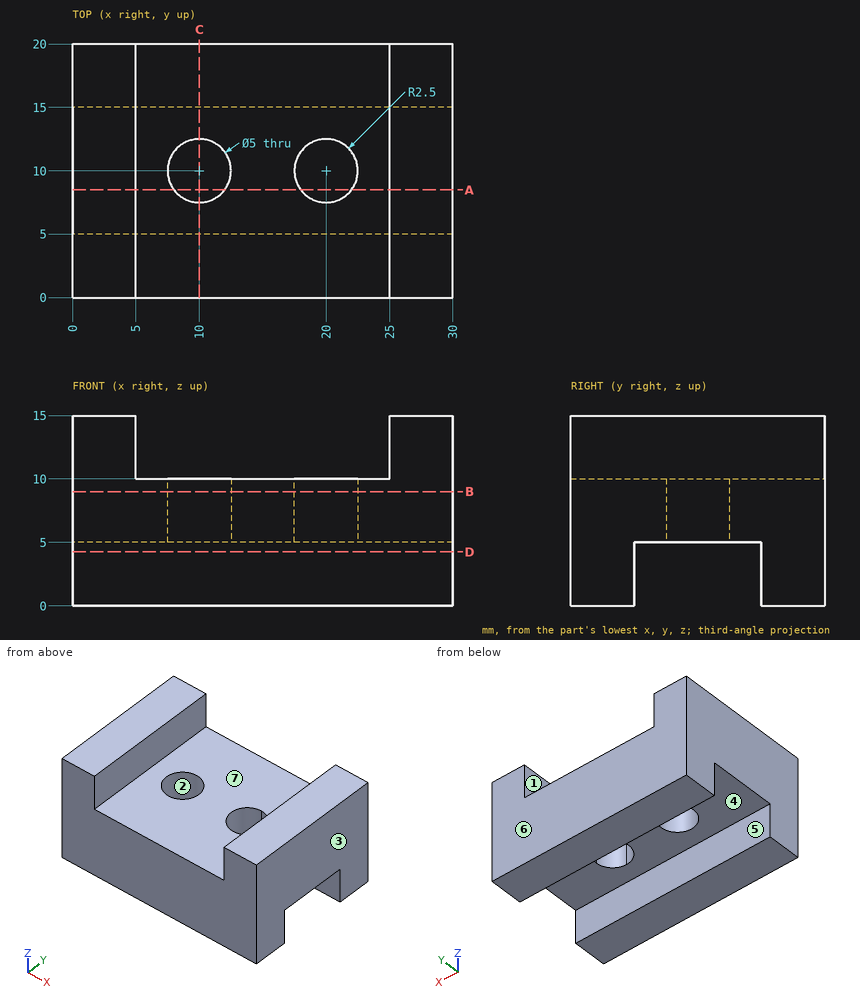
Geometry check sheet. Reference: drawing and pictorial views, mm from the part's lowest x, y, z. A direction names the side the tool comes from. Round coordinates to 2 decimals unless told otherwise and drop trailing zeros. Order: outer loops, then holes, each group sorted by start corner. A loop starts at its lowest first (then second) coordinate and runs counter-clockwise, first axis right, second up. Notation, with made-up numbers: (0, -26) - (38, -26) arc R19 cw to (38, -5) - close; hole circle Ø5 at (39.25, 48.25). An arc over 180 degrees is marked (long way). One line per question, with ' | ' between items. Start each with the question number.
(1) Depth check by flat-ended pin: pin 1 Ø5 at (x, y) = (10, 11) entering from +Z; pin 2 Ø8 at (x, y) = (12, 9.5) entering from -Z. Enter the tip coordinate at first touch or a pass-through.
(2) Access from +Z, -Z, +X, -X, +Y, -Y to the whole of each face (thin tool, end or side, straight path). Record for the marked faces 5, 6 and 7.
(3) Sectioned sample at D-D on z = 4.25. Record the cut outline in (x, y).
(4) Sectioned sample at B-B on z = 9. Record the cut outline in (x, y), and give its area (3 significant figures).
(5) Thickness scan on L1, parallel to Y at x = 13.75, z = 3.25; L2, parallel to Y at x = 10, z = 7.1; L3, parallel to X at y = 11.75, z = 9.5. Record the ranges inside material, lowest first. Write a range as [from, to].
(6) Sectioned sample at A-A on y = 8.5. Record the cut outline in (x, z), and give its area (3 significant figures).
(7) Sectioned sample at C-C on x = 10. Record the cut outline in (y, z), and give its area (3 significant figures).
(8) Release check for a two-part mould opening along X. For the marked faces 1, 2, 3 and 4 record: released by +X, released by -X, zero draft, split by the parting line, or undercut.
Conclusion:
1) pin 1: stops at z = 10 | pin 2: stops at z = 5
2) face 5: -Z, +X, -X | face 6: +Z, -Z, +X, -X, +Y | face 7: +Z, +Y, -Y
3) outline: (0, 0) - (30, 0) - (30, 5) - (0, 5) - close; (0, 15) - (30, 15) - (30, 20) - (0, 20) - close
4) outline: (0, 0) - (30, 0) - (30, 20) - (0, 20) - close; hole circle Ø5 at (10, 10); hole circle Ø5 at (20, 10) | area: 561 mm2
5) L1: y = [0, 5], [15, 20] | L2: y = [0, 7.5], [12.5, 20] | L3: x = [0, 8.21], [11.79, 18.21], [21.79, 30]
6) outline: (0, 5) - (8, 5) - (8, 10) - (5, 10) - (5, 15) - (0, 15) - close; (12, 5) - (18, 5) - (18, 10) - (12, 10) - close; (22, 5) - (30, 5) - (30, 15) - (25, 15) - (25, 10) - (22, 10) - close | area: 160 mm2
7) outline: (0, 0) - (5, 0) - (5, 5) - (7.5, 5) - (7.5, 10) - (0, 10) - close; (12.5, 5) - (15, 5) - (15, 0) - (20, 0) - (20, 10) - (12.5, 10) - close | area: 125 mm2
8) face 1: undercut | face 2: undercut | face 3: released by +X | face 4: zero draft
